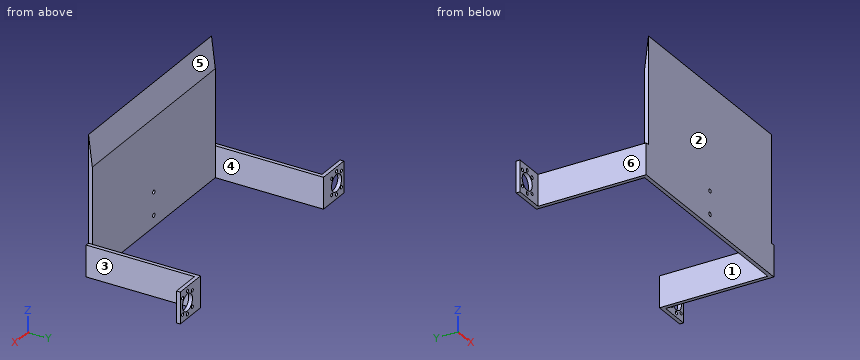
```python
from build123d import *

# Parameters (mm, degrees)
SKETCH1_W           = 454.914
SKETCH1_H           = 381
BOSS_EXTRUDE1_DEPTH = 187.96
SKETCH3_W           = 50.0126
SKETCH3_H           = 202.0062
CUT_EXTRUDE1_DEPTH  = 623.444141266
SKETCH4_R           = 14
CUT_EXTRUDE2_DEPTH  = 623.444141266
SKETCH5_W           = 342.1888
SKETCH5_H           = 381
CUT_EXTRUDE3_DEPTH  = 181.61
SKETCH6_W           = 178.9938
SKETCH6_H           = 181.597400076
CUT_EXTRUDE4_DEPTH  = 50.0126
SKETCH7_W           = 178.9938
SKETCH7_H           = 181.597400076
CUT_EXTRUDE5_DEPTH  = 50.0126
SKETCH10_W          = 202.0062
SKETCH10_H          = 187.96
CUT_EXTRUDE6_DEPTH  = 587.885938937
SKETCH11_R          = 2.7499945
SKETCH11_R_2        = 2.75
CUT_EXTRUDE7_DEPTH  = 623.444141266
SKETCH12_R          = 2.75
CUT_EXTRUDE8_DEPTH  = 623.444141266
BOSS_EXTRUDE2_DEPTH = 342.1888
SKETCH15_W          = 56.3626
SKETCH15_H          = 126.6698
CUT_EXTRUDE9_DEPTH  = 623.444141266
SKETCH16_R          = 3.175
CUT_EXTRUDE10_DEPTH = 623.444141266


with BuildPart() as part:
    # Sketch1 → Boss-Extrude1 (new body)
    with BuildSketch(Plane(origin=(0, 0, 0), x_dir=(1, 0, 0), z_dir=(0, 1, 0))):
        with Locations((227.457, 190.5)):
            Rectangle(SKETCH1_W, SKETCH1_H)
    extrude(amount=BOSS_EXTRUDE1_DEPTH)

    # Sketch3 → Cut-Extrude1 (cut, through all)
    with BuildSketch(Plane(origin=(0, 187.96, 0), x_dir=(1, 0, 0), z_dir=(0, 1, 0))):
        with Locations((429.9077, 101.0031)):
            Rectangle(SKETCH3_W, SKETCH3_H)
        with Locations((25.0063, 101.0031)):
            Rectangle(SKETCH3_W, SKETCH3_H)
    extrude(amount=-CUT_EXTRUDE1_DEPTH, mode=Mode.SUBTRACT)

    # Sketch4 → Cut-Extrude2 (cut, through all)
    with BuildSketch(Plane(origin=(0, 187.96, 0), x_dir=(1, 0, 0), z_dir=(0, 1, 0))):
        with Locations(Location((20.066, 355.092, 0), (0, 0, 270))):
            Circle(SKETCH4_R)
        with Locations(Location((434.848, 355.092, 0), (0, 0, 270))):
            Circle(SKETCH4_R)
    extrude(amount=-CUT_EXTRUDE2_DEPTH, mode=Mode.SUBTRACT)

    # Sketch5 → Cut-Extrude3 (cut)
    with BuildSketch(Plane(origin=(0, 187.96, 0), x_dir=(1, 0, 0), z_dir=(0, 1, 0))):
        with Locations((227.457, 190.5)):
            Rectangle(SKETCH5_W, SKETCH5_H)
    extrude(amount=-CUT_EXTRUDE3_DEPTH, mode=Mode.SUBTRACT)

    # Sketch6 → Cut-Extrude4 (cut)
    with BuildSketch(Plane(origin=(454.914, 0, 0), x_dir=(0, 0, -1), z_dir=(1, 0, 0))):
        with Locations((291.5031, 90.798700038)):
            Rectangle(SKETCH6_W, SKETCH6_H)
    extrude(amount=-CUT_EXTRUDE4_DEPTH, mode=Mode.SUBTRACT)

    # Sketch7 → Cut-Extrude5 (cut)
    with BuildSketch(Plane.ZY):
        with Locations((-291.5031, 90.798700038)):
            Rectangle(SKETCH7_W, SKETCH7_H)
    extrude(amount=-CUT_EXTRUDE5_DEPTH, mode=Mode.SUBTRACT)

    # Sketch10 → Cut-Extrude6 (cut, through all)
    with BuildSketch(Plane(origin=(404.9014, 0, 0), x_dir=(0, 0, -1), z_dir=(1, 0, 0))):
        with Locations((101.0031, 93.98)):
            Rectangle(SKETCH10_W, SKETCH10_H)
    extrude(amount=-CUT_EXTRUDE6_DEPTH, mode=Mode.SUBTRACT)

    # Sketch11 → Cut-Extrude7 (cut, through all)
    with BuildSketch(Plane(origin=(0, 187.96, 0), x_dir=(1, 0, 0), z_dir=(0, 1, 0))):
        with Locations(Location((434.848, 374.174211985, 0), (0, 0, 270))):
            Circle(SKETCH11_R)
        with Locations(Location((448.283028843, 368.609240827, 0), (0, 0, 270))):
            Circle(SKETCH11_R_2)
        with Locations(Location((421.412971157, 368.609240827, 0), (0, 0, 270))):
            Circle(SKETCH11_R_2)
        with Locations(Location((448.283028843, 341.739183142, 0), (0, 0, 270))):
            Circle(SKETCH11_R_2)
        with Locations(Location((434.848, 336.174211985, 0), (0, 0, 270))):
            Circle(SKETCH11_R_2)
        with Locations(Location((421.412971157, 341.739183142, 0), (0, 0, 270))):
            Circle(SKETCH11_R_2)
    extrude(amount=-CUT_EXTRUDE7_DEPTH, mode=Mode.SUBTRACT)

    # Sketch12 → Cut-Extrude8 (cut, through all)
    with BuildSketch(Plane(origin=(0, 187.96, 0), x_dir=(1, 0, 0), z_dir=(0, 1, 0))):
        with Locations(Location((20.066, 374.092, 0), (0, 0, 270))):
            Circle(SKETCH12_R)
        with Locations(Location((6.630971157, 368.527028843, 0), (0, 0, 270))):
            Circle(SKETCH12_R)
        with Locations(Location((33.501028843, 368.527028843, 0), (0, 0, 270))):
            Circle(SKETCH12_R)
        with Locations(Location((33.501028843, 341.656971157, 0), (0, 0, 270))):
            Circle(SKETCH12_R)
        with Locations(Location((20.066, 336.092, 0), (0, 0, 270))):
            Circle(SKETCH12_R)
        with Locations(Location((6.630971157, 341.656971157, 0), (0, 0, 270))):
            Circle(SKETCH12_R)
    extrude(amount=-CUT_EXTRUDE8_DEPTH, mode=Mode.SUBTRACT)

    # Sketch13 → Boss-Extrude2 (add)
    with BuildSketch(Plane(origin=(398.5514, 0, 0), x_dir=(0, 0, -1), z_dir=(1, 0, 0))):
        Polygon((202.0062, 0), (150.289600182, 0), (202.0062, 6.35), align=None)
    extrude(amount=-BOSS_EXTRUDE2_DEPTH)

    # Sketch15 → Cut-Extrude9 (cut, through all)
    with BuildSketch(Plane(origin=(0, 187.96, 0), x_dir=(1, 0, 0), z_dir=(0, 1, 0))):
        with Locations((426.7327, 265.3411)):
            Rectangle(SKETCH15_W, SKETCH15_H)
        with Locations((28.1813, 265.3411)):
            Rectangle(SKETCH15_W, SKETCH15_H)
    extrude(amount=-CUT_EXTRUDE9_DEPTH, mode=Mode.SUBTRACT)

    # Sketch16 → Cut-Extrude10 (cut, through all)
    with BuildSketch(Plane.XZ):
        with Locations(Location((227.457, -361.95, 0), (0, 0, 270))):
            Circle(SKETCH16_R)
        with Locations(Location((227.457, -323.85, 0), (0, 0, 270))):
            Circle(SKETCH16_R)
    extrude(amount=-CUT_EXTRUDE10_DEPTH, mode=Mode.SUBTRACT)


solid = part.part
```
Input: part model. Units: mm. Frame: model coordinates. Face numbers are marked on the shaded views. A direction names the side the tool comes from. Give positions to 0.01 mm unless a question says otherwise; leave off trailing zeros. Order: outer loops, then holes, each group sorted by start corner. A loop starts at its lowest first (then second) coordinate and runs counter-clockwise, first axis right, second up.
1. Material intervals for L1, parallel to X at y = 80, z = -346; L2, parallel to Y at x = 60.5, z = -311.5; L3, parallel to Z at x = 401.5, y = 22, sorted ascending.
Derived:
L1: x = 50.01 to 56.36, 398.55 to 404.9
L2: y = 0 to 6.35
L3: z = -381 to -328.68
2. Section B-B on x = 110. Return the cut outline in (y, z).
Derived:
outline: (0, -381) - (6.35, -381) - (6.35, -202.01) - (0, -150.29) - close
3. Mould query, pull axis X, two halves, no side actions, for the marked faces 4, 5 and 6. Classes: released by +X, released by -X, zero draft, split by the parting line, or undercut.
Derived:
face 4: undercut
face 5: zero draft
face 6: released by -X
4. Section C-C on z = -269. Return the cut outline in (x, y).
Derived:
outline: (56.36, 0) - (398.55, 0) - (398.55, 6.35) - (56.36, 6.35) - close
5. Reachability of the marked faces 1, 2 and 3 from +Z, -Z, +X, -X, +Y, -Y: full face, straight path, thin tool, end or side. Return the list, or none.
Derived:
face 1: +Z, -Z, +Y
face 2: +Z, -Z, +X, -X, -Y
face 3: +Z, -Z, +X, -Y
6. Pin query (flat end, axial travel): pin 1 (5 mm diameter, centred on x = 397.5, z = -251, fed in from +Y); pin 2 (15.5 mm diameter, centred on y = 133, z = -346, fed in from +X); pin 3 (7 mm diameter, centred on x = 6.63, z = -341.66, fed in from -Y); pin 4 (3.5 mm diameter, centred on x = 448.28, z = -341.74, fed in from -Y). Return the tip coordinate at first contact, or that it passes through.
Derived:
pin 1: stops at y = 6.35
pin 2: stops at x = 404.9
pin 3: stops at y = 181.6
pin 4: passes through
7. Section A-A on y = 147.5. Return the cut outline in (x, z), and give its area (3 significant figures).
Derived:
outline: (50.01, -381) - (56.36, -381) - (56.36, -328.68) - (50.01, -328.68) - close; (398.55, -381) - (404.9, -381) - (404.9, -328.68) - (398.55, -328.68) - close
area: 665 mm2
